Here's how the part is built. I have some questions about the finished solid (model axes, mm). Coordinates: 2 decimals unless noted, no trailing zeros. Write each loop counter-clockwise with the first axis right and the second up, starting at its lowest first coordinate (ties: lowest second). Pieces come first, ordered by that corner, then holes.
```python
from build123d import *

# Parameters (mm, degrees)
F2_DEPTH = 3.6
F4_DEPTH = 3.6
F5_W     = 20.3048
F5_H     = 1.8
F6_DEPTH = 1.8
F7_R     = 2.376
F8_R     = 0.5


with BuildPart() as f2:
    # F1 (on Top) → F2 (new body)
    with BuildSketch(Plane.XY):
        with BuildLine():
            Line((-10.1524, -54.15), (10.1524, -54.15))
            ThreePointArc((10.1524, -54.15), (14.3933436308, -52.3933436308), (16.15, -48.1524))
            Line((16.15, -48.1524), (16.15, 48.1524))
            ThreePointArc((16.15, 48.1524), (14.3933436308, 52.3933436308), (10.1524, 54.15))
            Line((10.1524, 54.15), (-10.1524, 54.15))
            ThreePointArc((-10.1524, 54.15), (-14.3933436308, 52.3933436308), (-16.15, 48.1524))
            Line((-16.15, 48.1524), (-16.15, -48.1524))
            ThreePointArc((-16.15, -48.1524), (-14.3933436308, -52.3933436308), (-10.1524, -54.15))
        make_face()
    extrude(amount=F2_DEPTH)

    # F3 (on face) → F4 (join)
    with BuildSketch(Plane.XZ.offset(54.15)):
        Polygon((9, 3.6), (-9, 3.6), (-9, 1.8), (-9, 0), (9, 0), (9, 1.8), align=None)
    extrude(amount=F4_DEPTH)

    # F5 (on face) → F6 (join)
    with BuildSketch(Plane(origin=(0, 54.15, 0), x_dir=(-1, 0, 0), z_dir=(0, 1, 0))):
        with Locations((0, 0.9)):
            Rectangle(F5_W, F5_H)
    extrude(amount=F6_DEPTH)

    # F7
    f7_edges = [f2.edges().sort_by_distance(p)[0] for p in [
        (0, -57.75, 3.6),
    ]]
    fillet(f7_edges, radius=F7_R)

    # F8
    f8_edges = [f2.edges().sort_by_distance(p)[0] for p in [
        (0, 55.95, 1.8),
    ]]
    fillet(f8_edges, radius=F8_R)


solid = f2.part
```
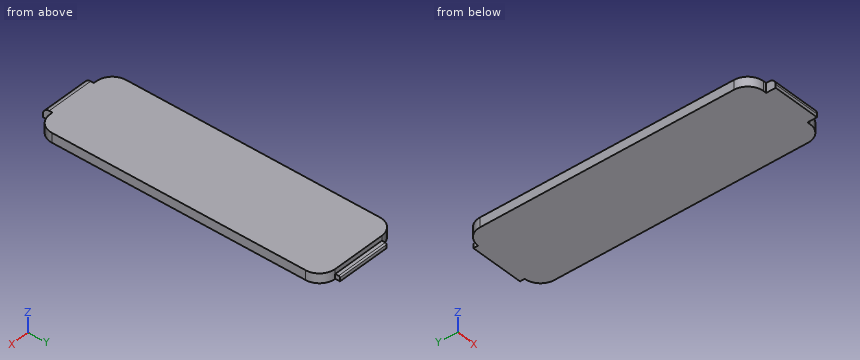
1) Imagine slicing it at A-A on z = 2.6. Please give me the cut outline in (x, y).
Values follow:
outline: (-16.15, -48.15) arc R6 ccw to (-10.15, -54.15) - (-9, -54.15) - (-9, -57.31) - (9, -57.31) - (9, -54.15) - (10.15, -54.15) arc R6 ccw to (16.15, -48.15) - (16.15, 48.15) arc R6 ccw to (10.15, 54.15) - (-10.15, 54.15) arc R6 ccw to (-16.15, 48.15) - close
2) Imagine slicing it at B-B on x = -13.5. Please give me the cut outline in (y, z), then the cut area to 3 significant figures.
Values follow:
outline: (-53.13, 0) - (53.13, 0) - (53.13, 3.6) - (-53.13, 3.6) - close
area: 383 mm2
3) I need wall thicknesses on probe 1 along Y at (x, z) = (6, 3.3); probe 2 along Y at (x, z) = (-13.5, 1.45); probe 3 along X at (y, z) = (50, 3.3). Which ranges of each line are inside material? Lowest first, please.
Values follow:
probe 1: y = -56.53 to 54.15
probe 2: y = -53.13 to 53.13
probe 3: x = -15.86 to 15.86
4) Will these pins go through, and if not, where does the flat tip stop? pin 1 (2 mm diameter, centred on y = 55.5, z = 1, fed in from -X); pin 2 (0.9 mm diameter, centred on x = 9.5, z = 2.5, fed in from -Y); pin 3 (1.5 mm diameter, centred on x = 9.5, z = 2, fed in from -Y).
Values follow:
pin 1: stops at x = -10.15
pin 2: stops at y = -54.15
pin 3: stops at y = -57.74
